Source: CAD feature listing. Evaluate the final solid. Frame: model axes, mm. A direction names the side the tool comes from. Give positions to 0.01 mm unless a question says otherwise; leave off trailing zeros. Loops run counter-clockwise (first coordinate to the right, second up) from the corner with the lowest first, then second, coordinate; pieces in that order, holes last. Notation, with made-up numbers: (-39.5, 43.25) - (-18.5, 43.25) arc R29 cw to (-18.5, 70.25) - close; hole circle Ø3 at (35, -7). An arc over 180 degrees is marked (long way). Put each result on its own line as item: value.
```python
from build123d import *

# Parameters (mm, degrees)
F1_DEPTH = 7
F2_R     = 1.5
F3_R     = 1.8


with BuildPart() as f1:
    # F0 (on Right) → F1 (new body)
    with BuildSketch(Plane.YZ):
        Polygon((-40.4, 35), (-41, 35), (-41, -35), (41, -35), (41, 35), (40.4, 35), (40.4, -34.4), (-40.4, -34.4), align=None)
    extrude(amount=F1_DEPTH)

    # F2
    f2_edges = [f1.edges().sort_by_distance(p)[0] for p in [
        (3.5, -40.4, -34.4),
        (3.5, 40.4, -34.4),
    ]]
    fillet(f2_edges, radius=F2_R)

    # F3
    f3_edges = [f1.edges().sort_by_distance(p)[0] for p in [
        (3.5, -41, -35),
        (3.5, 41, -35),
    ]]
    fillet(f3_edges, radius=F3_R)


solid = f1.part
```
1) Mould query, pull axis Y, two halves, no side actions, for faces 1 (the cylindrical face through (3.549, -40.459, -34.487)), 2 (the flat face through (3, 40.4, 2)), 3 (the flat face through (3, 41, 0)). Classes: pulls with the +Y half, pulls with the -Y half, needs draft (parallel to the pull), parting line crosses it, or undercut.
Check result:
face 1: pulls with the -Y half
face 2: undercut
face 3: pulls with the +Y half
2) Section query B-B, the plane x = 1.5. Output: boundary loops of the cut face in (y, z).
Check result:
outline: (-41, -33.2) arc R1.8 ccw to (-39.2, -35) - (39.2, -35) arc R1.8 ccw to (41, -33.2) - (41, 35) - (40.4, 35) - (40.4, -32.9) arc R1.5 cw to (38.9, -34.4) - (-38.9, -34.4) arc R1.5 cw to (-40.4, -32.9) - (-40.4, 35) - (-41, 35) - close
3) Material intervals for line 1 along Y through (x, z) = (0.75, -32); line 2 along Z through (x, y) = (5.25, 13), sorted ascending. Write a range as [from, to].
Check result:
line 1: [-41, -40.4], [40.4, 41]
line 2: [-35, -34.4]
4) Pin query (flat end, axial travel): P1, Ø2, axis at x = 5, y = -18.5, coming from the +Z side. Return the tip coordinate at first contact, or that it passes through.
Check result:
P1: z = -34.4
5) Access query for faces 4 (the flat face through (3, -41, 1)), 5 (the flat face through (3, 1, -34.4)). Directions: +Z, -Z, +X, -X, +Y, -Y. A direction counts if a zero-diameter tool reaches every point of the face in a straight line with its end or side. Return the directions, or none.
Check result:
face 4: +Z, -Z, +X, -X, -Y
face 5: +Z, +X, -X
6) Section query C-C, the plane y = 22. Output: boundary loops of the cut face in (x, z).
Check result:
outline: (0, -35) - (7, -35) - (7, -34.4) - (0, -34.4) - close
7) Section query A-A, the plane z = -26. Output: boundary loops of the cut face in (x, y).
Check result:
outline: (0, -41) - (7, -41) - (7, -40.4) - (0, -40.4) - close; (0, 40.4) - (7, 40.4) - (7, 41) - (0, 41) - close
